Can you work these out from the model? Positions are in its coordinate system, mm. A direction names the side the tool comes from. Coordinates: 2 decimals unless noted, no trailing zeros. Order: outer loops, then holes, each group sorted by start corner. A loop starts at its lowest first (then second) coordinate and runs counter-clockwise, first axis right, second up. Notation, with made-up numbers: (-0.75, 44) - (51.25, 44) arc R28 cw to (51.25, 72) - close; hole circle Ø10 at (71, -12.5). An arc over 180 degrees is marked (long way). Use a Markdown table: item, result. Add a question column.
(1) For pin 1 Ø1.5 at (y, z) = (-1, 3) entering from +X, with a flat end and sliding along its axis, tell me the tip position at first contact or that it passes through.
(2) I want a section at C-C (z = 4.5). List the corners of the cut face in (x, y) for me, and give its area (3 significant figures).
(3) On a 3-axis mill with a long thin cutter (end or side, diameter ignored), from which of +Z, -Z, +X, -X, +Y, -Y can I reach the whole of each face in a straight line? I mean faces 1 (the cylindrical face through (-1.437, 1.318, 4.958)), 2 (the flat face through (0, 0, 0)). Say none if no direction works.
(4) I want a section at A-A (y = 0). List the corners of the cut face in (x, z) for me, and give its area (3 significant figures).
(5) I want a section at D-D (z = 1.5). List the corners of the cut face in (x, y) for me, and give its area (3 significant figures).
(6) If I drill on L1, parallel to Y at x = -0.1, z = 2.5; L2, parallel to Z at x = 0.2, y = -2; L3, parallel to X at y = -1.3, z = 2.5, over which ranges is the centre line in solid material (lowest first)? Write a range as [from, to].
```python
from build123d import *

# Parameters (mm, degrees)
SKETCH_1_R      = 2.4
EXTRUDE_1_DEPTH = 2
SKETCH_2_R      = 1.95
EXTRUDE_2_DEPTH = 6
CHAMFER_1_SIZE  = 0.25


with BuildPart() as part:
    # 草图1 → 拉伸1 (new body)
    with BuildSketch(Plane.XY):
        Circle(SKETCH_1_R)
    extrude(amount=EXTRUDE_1_DEPTH)

    # 草图2 → 拉伸2 (add)
    with BuildSketch(Plane.XY.offset(2)):
        Circle(SKETCH_2_R)
    extrude(amount=EXTRUDE_2_DEPTH)

    # 倒角1
    chamfer_1_edges = [part.edges().sort_by_distance(p)[0] for p in [
        (-2.4, 0, 2),
    ]]
    chamfer(chamfer_1_edges, length=CHAMFER_1_SIZE)


solid = part.part
```
Answers follow:
| question | item | result |
|---|---|---|
| 1 | pin 1 | stops at x = 1.93 |
| 2 | outline | circle Ø3.9 at (0, 0) |
| 2 | area | 11.9 mm² |
| 3 | face 1 | +Z |
| 3 | face 2 | -Z, +X, -X, +Y, -Y |
| 4 | outline | (-2.4, 0) - (2.4, 0) - (2.4, 1.75) - (2.15, 2) - (1.95, 2) - (1.95, 8) - (-1.95, 8) - (-1.95, 2) - (-2.15, 2) - (-2.4, 1.75) - close |
| 4 | area | 32.9 mm² |
| 5 | outline | circle Ø4.8 at (0, 0) |
| 5 | area | 18.1 mm² |
| 6 | L1 | y = [-1.95, 1.95] |
| 6 | L2 | z = [0, 2] |
| 6 | L3 | x = [-1.45, 1.45] |
